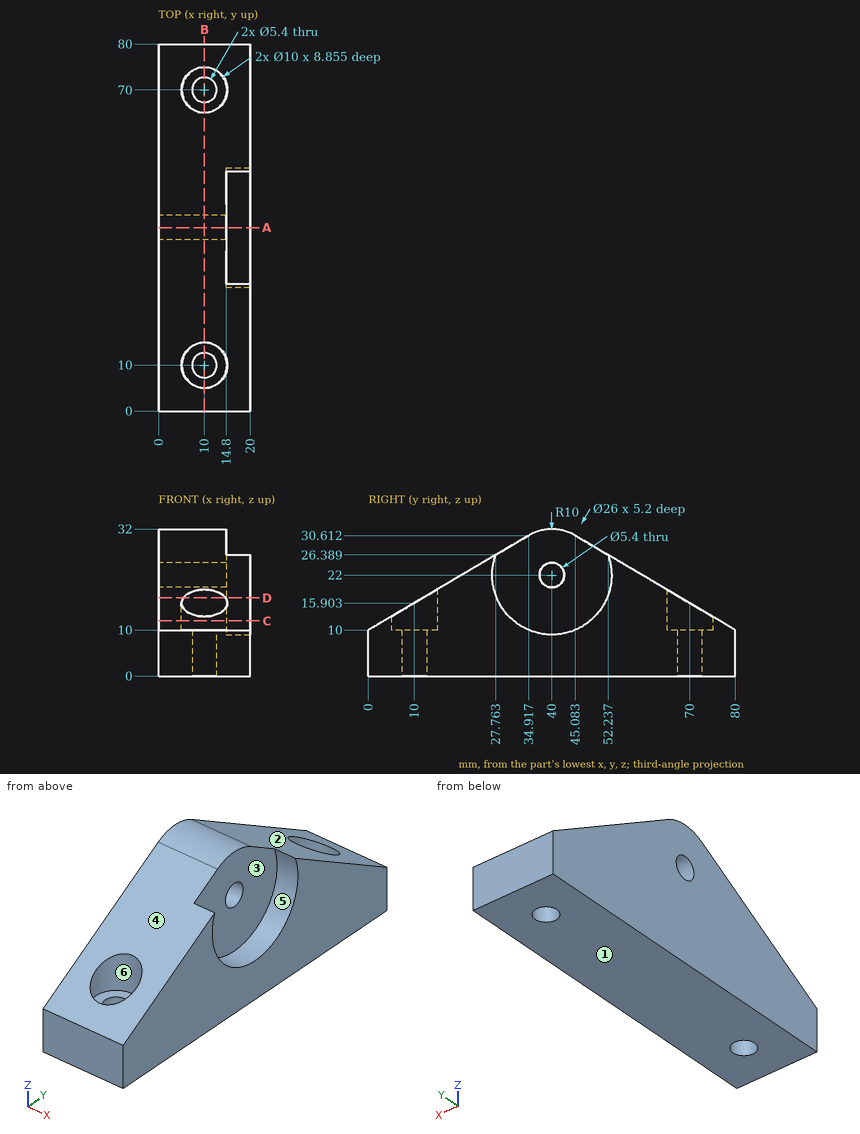
Part print with two shaded views. Sizes in mm from the minimum x, y, z corner. A direction names the side the tool comes from. Give positions to 0.01 mm unless a question says otherwise; leave off trailing zeros. Write each loop counter-clockwise with the first axis right and the second up, starting at its lowest first coordinate (ties: lowest second). Pieces come first, ordered by that corner, then holes.
1) Pin check, flat tips, straight feed: pin 1 (4 mm diameter, centred on x = 17, y = 55.5, fed in from +Z); pin 2 (6 mm diameter, centred on y = 39.5, z = 20.5, fed in from +X); pin 3 (8 mm diameter, centred on x = 3, z = 19, fed in from +Y). Stop position of each tip, or through.
Resolved:
pin 1: stops at z = 25.64
pin 2: stops at x = 14.8
pin 3: stops at y = 71.53
2) Probe L1, parallel to Y at x = 10, z = 4.5; L2, parallel to X at y = 70, z = 12.5; L3, parallel to X at y = 31, z = 17. List the from-to ranges inside material, lowest first.
Resolved:
L1: y = 0 to 7.3, 12.7 to 67.3, 72.7 to 80
L2: x = 0 to 5, 15 to 20
L3: x = 0 to 14.8
3) Which spindle directions (+Z, -Z, +X, -X, +Y, -Y) get a long thin tool onto all of the face, cutting with end or side? Do the marked faces 4, 5 and 6. Say none if no direction does.
Resolved:
face 4: +Z, +X, -X, -Y
face 5: +X
face 6: +Z
4) Cut at A-A on y = 40. Write the cut outline in (x, z).
Resolved:
outline: (0, 0) - (20, 0) - (20, 9) - (14.8, 9) - (14.8, 19.3) - (0, 19.3) - close; (0, 24.7) - (14.8, 24.7) - (14.8, 32) - (0, 32) - close
5) Two-plate mould, pull along Y, no slides. Class the marked faces 1, 2 and 3: released by +Y, released by -Y, zero draft, split by the parting line, or undercut.
Resolved:
face 1: zero draft
face 2: released by +Y
face 3: undercut
6) Cut at D-D on z = 17. Write the cut outline in (x, y).
Resolved:
outline: (0, 11.86) - (5.36, 11.86) arc R5 cw to (14.64, 11.86) - (20, 11.86) - (20, 28) - (14.8, 28) - (14.8, 52) - (20, 52) - (20, 68.14) - (14.64, 68.14) arc R5 cw to (5.36, 68.14) - (0, 68.14) - close
7) Cut at B-B on x = 10. Write the cut outline in (y, z) (1 decimal).
Resolved:
outline: (0, 0) - (7.3, 0) - (7.3, 10) - (5, 10) - (5, 13) - (0, 10) - close; (12.7, 0) - (67.3, 0) - (67.3, 10) - (65, 10) - (65, 18.9) - (45.1, 30.6) arc R10 ccw to (34.9, 30.6) - (15, 18.9) - (15, 10) - (12.7, 10) - close; (72.7, 0) - (80, 0) - (80, 10) - (75, 13) - (75, 10) - (72.7, 10) - close; hole circle Ø5.4 at (40, 22)
8) Cut at C-C on z = 12. Write the cut outline in (x, y), then the cut area to 3 significant figures.
Resolved:
outline: (0, 3.39) - (20, 3.39) - (20, 31.69) - (14.8, 31.69) - (14.8, 48.31) - (20, 48.31) - (20, 76.61) - (0, 76.61) - close; hole circle Ø10 at (10, 10); hole circle Ø10 at (10, 70)
area: 1,220 mm2
